```python
from build123d import *

# Parameters (mm, degrees)
F1_DEPTH = 10
F0_R     = 9
F2_DEPTH = 1.25
F3_R     = 0.5


with BuildPart() as f1:
    # F0 (on Top) → F1 (new body)
    with BuildSketch(Plane.XY):
        Polygon((-7.207986, 0.779381), (-4.278957, -5.852609), (2.92903, -6.63199), (7.207986, -0.779381), (4.278957, 5.852609), (-2.92903, 6.63199), align=None)
        with BuildLine():
            ThreePointArc((2.05, 1.679286), (2.495496, 0.891628), (2.65, 0))
            ThreePointArc((2.65, 0), (2.495496, -0.891628), (2.05, -1.679286))
            ThreePointArc((2.05, -1.679286), (-0.891628, -2.495496), (-2.65, 0))
            ThreePointArc((-2.65, 0), (-0.891628, 2.495496), (2.05, 1.679286))
        make_face(mode=Mode.SUBTRACT)
        with BuildLine():
            ThreePointArc((2.05, -1.679286), (2.495496, -0.891628), (2.65, 0))
            ThreePointArc((2.65, 0), (2.495496, 0.891628), (2.05, 1.679286))
            Line((2.05, 1.679286), (2.05, 0))
            Line((2.05, 0), (2.05, -1.679286))
        make_face()
    extrude(amount=F1_DEPTH)

    # F0 (on Top) → F2 (join)
    with BuildSketch(Plane.XY):
        Circle(F0_R)
        Polygon((2.92903, -6.63199), (-4.278957, -5.852609), (-7.207986, 0.779381), (-2.92903, 6.63199), (4.278957, 5.852609), (7.207986, -0.779381), align=None, mode=Mode.SUBTRACT)
    extrude(amount=F2_DEPTH)

    # F3
    f3_edges = [f1.edges().sort_by_distance(p)[0] for p in [
        (-0.674963, -6.242299, 10),
        (5.068508, -3.705685, 10),
        (5.743471, 2.536614, 10),
        (0.674963, 6.242299, 10),
        (-5.068508, 3.705685, 10),
        (-5.743471, -2.536614, 10),
    ]]
    fillet(f3_edges, radius=F3_R)


solid = f1.part
```
Work out the finished part from the listing and answer in its coordinate system (mm). A direction names the side the tool comes from. Round coordinates to 2 decimals unless told otherwise and drop trailing zeros. Write each loop counter-clockwise with the first axis right and the second up, starting at its lowest first coordinate (ties: lowest second). Pieces come first, ordered by that corner, then holes. Notation, with made-up numbers: (77.25, 59.5) -> (109.25, 59.5) arc R25 cw to (109.25, 83.5) -> close; hole circle Ø8 at (75.25, 17). An arc over 180 degrees is marked (long way). Write each question's results on one line, items separated by ' | '.
1) The part is cut by section B-B (z = 9.75). Write down the section's boundary in (x, y).
Findings:
outline: (-7.13, 0.77) -> (-4.23, -5.79) -> (2.9, -6.56) -> (7.13, -0.77) -> (4.23, 5.79) -> (-2.9, 6.56) -> close; hole (2.05, -1.68) -> (2.05, 1.68) arc R2.65 ccw (long way) to start
2) Consider line 1 along Z through (x, y) = (-4, -8); line 2 along X through (y, z) = (0, 3.5); line 3 along Y through (x, z) = (-1.25, 9.75). Determine where each line is inside the solid, lowest interval first. Write a range as [from, to].
Findings:
line 1: z = [0, 1.25] | line 2: x = [-6.86, -2.65], [2.05, 6.86] | line 3: y = [-6.11, -2.34], [2.34, 6.38]
3) For a pull along Y with two mould halves and no side action, classify faces 6 (the cylindrical face through (-0.609, -6.106, 9.85)), 7 (the flat face through (2.05, 0, 5)), 8 (the flat face through (-5.039, 3.747, 5.317)) as +Y half, -Y half, draft (parallel to the pull), parting line (faces both ways), or undercut.
Findings:
face 6: -Y half | face 7: undercut | face 8: +Y half
4) Flat-ended cylindrical pins translate along their axes: pin 1 (3.5 mm diameter, centred on y = 0.5, z = 4.5, fed in from -X); pin 2 (4 mm diameter, centred on x = 4.5, z = 2, fed in from -Y); pin 3 (6 mm diameter, centred on y = 2, z = 1.5, fed in from -X); pin 4 (4 mm diameter, centred on x = 5, z = 7, fed in from +Y). Find the tip coordinate at first contact, or state that the pin passes through.
Findings:
pin 1: stops at x = -7.21 | pin 2: stops at y = -8.6 | pin 3: stops at x = -9 | pin 4: stops at y = 5.99
5) Which of the six approach directions +Z, -Z, +X, -X, +Y, -Y give full straight-line access (tool end or side, diameter ignored) to faces 1 (the flat face through (-0.725, -6.237, 5.317)), 2 (the flat face through (4, -6, 1.25)), 3 (the flat face through (5.039, -3.747, 5.317)), 4 (the flat face through (5.764, 2.49, 5.317)), 5 (the cylindrical face through (-4.98, 3.58, 9.85))?
Findings:
face 1: +Z, -X, -Y | face 2: +Z | face 3: +Z, +X, -Y | face 4: +Z, +X, +Y | face 5: +Z, -X, +Y
6) The part is cut by section A-A (z = 5). Write down the section's boundary in (x, y).
Findings:
outline: (-7.21, 0.78) -> (-4.28, -5.85) -> (2.93, -6.63) -> (7.21, -0.78) -> (4.28, 5.85) -> (-2.93, 6.63) -> close; hole (2.05, -1.68) -> (2.05, 1.68) arc R2.65 ccw (long way) to start
